The listing builds one solid part. Answer for the finished solid, in the listing's coordinates (mm). A direction names the side the tool comes from. Coordinates: 2 decimals unless noted, no trailing zeros. Use a Markdown table: item, result. Add a question column.
Item 1: The mould has two halves that part along X. Classify faces 1 (the flat face through (-2, -0.27, -0.2)), 2 (the cylindrical face through (-5.86, 7.07, -0.42)), 3 (the flat face through (1, 0, 0)): released by +X, released by -X, zero draft, split by the parting line, or undercut.
Item 2: For faces 4 (the flat face through (-2.5, 0.162, 0)), 5 (the flat face through (-10.679, 14.046, -0.007)), determine the directions among +Z, -Z, +X, -X, +Y, -Y from which every point of the face is accessible in a straight line to the end or side of a thin tool.
Item 3: Flat-ended cylindrical pins translate along their axes: P1, Ø2, axis at x = -6.5, z = -1, coming from the +Y side; P2, Ø0.7, axis at x = -2.5, z = 0, coming from the -Y side; P3, Ø3, axis at y = 11.5, z = 0, coming from the -X side. Find the tip coordinate at first contact, or state that the pin passes through.
Item 4: Find the intervals of material crossed by line 1 along X through (y, z) = (-0.75, 2.25); line 2 along Y through (x, z) = (-0.5, 1.25); line 3 along Z through (x, y) = (-0.75, -1.25), in increasing order.
from build123d import *

# Parameters (mm, degrees)
Y_KSEKLIK_EKSTR_ZYON1_DEPTH      = 1
Y_KSEKLIK_EKSTR_ZYON1_DEPTH_BACK = 1
IZIM1_R                          = 3.5
RADYUS1_R                        = 1
RADYUS2_R                        = 1
IZIM2_W                          = 0.864396699
IZIM2_H                          = 0.432198349
Y_KSEKLIK_EKSTR_ZYON2_DEPTH      = 2


with BuildPart() as part:
    # Çizim1 → Yükseklik-Ekstrüzyon1 (new, two sides: drawn at the far end of the back side and taken through both)
    with BuildSketch(Plane(origin=(0, 0, 0), x_dir=(0, 0, -1), z_dir=(1, 0, 0)).offset(-Y_KSEKLIK_EKSTR_ZYON1_DEPTH_BACK)):
        Circle(IZIM1_R)
    extrude(amount=Y_KSEKLIK_EKSTR_ZYON1_DEPTH + Y_KSEKLIK_EKSTR_ZYON1_DEPTH_BACK)

    # Radyus1
    radyus1_edges = [part.edges().sort_by_distance(p)[0] for p in [
        (1, 0, 3.5),
    ]]
    fillet(radyus1_edges, radius=RADYUS1_R - 0.0001)  # a hair under: the kernel refuses the full size

    # Radyus2
    radyus2_edges = [part.edges().sort_by_distance(p)[0] for p in [
        (-1, 0, 3.5),
    ]]
    fillet(radyus2_edges, radius=RADYUS2_R - 0.0001)  # a hair under: the kernel refuses the full size

    # Çizim2 → Yükseklik-Ekstrüzyon2 (add)
    with BuildSketch(Plane.ZY.offset(1)):
        with Locations((0.009004132, -0.054024793)):
            Rectangle(IZIM2_W, IZIM2_H)
    extrude(amount=Y_KSEKLIK_EKSTR_ZYON2_DEPTH)

    # Çizim3 → Döndür-İnce1 (revolve)
    with BuildSketch(Plane.XY, mode=Mode.PRIVATE) as d_nd_r_nce1_sk:
        Polygon((-1.61474818, 0), (-10.685328889, 14.04226294), (-11.105326504, 13.77096605), (-2.034745795, -0.27129689), align=None)
    revolve(d_nd_r_nce1_sk.sketch.rotate(Axis((-1.61474818, 0, 0), (-0.5425937809668819, 0.8399952314484074, 0)), 180), axis=Axis((-1.61474818, 0, 0), (-0.5425937809668819, 0.8399952314484074, 0)))

    # Çizim4 → Döndür-İnce2 (revolve)
    with BuildSketch(Plane.XY, mode=Mode.PRIVATE) as d_nd_r_nce2_sk:
        Polygon((-2.810513045, 0), (-11.199411855, 5.686357854), (-11.367738433, 5.438031127), (-2.978839623, -0.248326726), align=None)
    revolve(d_nd_r_nce2_sk.sketch.rotate(Axis((-2.810513045, 0, 0), (-0.8277557549139161, 0.561088593901973, 0)), 180), axis=Axis((-2.810513045, 0, 0), (-0.8277557549139161, 0.561088593901973, 0)))


solid = part.part
Solution:
| question | item | result |
|---|---|---|
| 1 | face 1 | zero draft |
| 1 | face 2 | undercut |
| 1 | face 3 | released by +X |
| 2 | face 4 | none |
| 2 | face 5 | +Z, -Z, -X, +Y |
| 3 | P1 | stops at y = 9.41 |
| 3 | P2 | stops at y = -0.27 |
| 3 | P3 | stops at x = -10.61 |
| 4 | line 1 | x = -1 to 1 |
| 4 | line 2 | y = -3.13 to 3.13 |
| 4 | line 3 | z = -2.9 to 2.9 |
